Autodesk Inventor part; units mm, degrees
ref_plane "YZ Plane" through (0, 0, 0) normal (1, 0, 0) x (0, 1, 0)
ref_plane "XZ Plane" through (0, 0, 0) normal (0, 1, 0) x (-1, 0, 0)
ref_plane "XY Plane" through (0, 0, 0) normal (0, 0, 1) x (1, 0, 0)
sketch "Sketch1" plane through (0, 0, 0) normal (0, 0, 1) x (1, 0, 0)
  line L0 (323.3438, -62.5) -> (393.7095, -62.5)
  arc A0 (323.3438, -62.5) -> (278.3438, -107.5) centre (323.3438, -107.5) ccw
  line L1 (278.3438, -115) -> (278.3438, -107.5)
  arc A1 (273.3438, -120) -> (278.3438, -115) centre (273.3438, -115) ccw
  line L2 (149.8438, -120) -> (273.3438, -120)
  arc A2 (442.4011, -101.1364) -> (393.7095, -62.5) centre (393.7095, -112.5) ccw
  arc A3 (442.4011, -101.1364) -> (447.2702, -105) centre (447.2702, -100) ccw
  line L3 (453.1438, -105) -> (447.2702, -105)
  arc A4 (453.1438, -105) -> (468.1438, -90) centre (453.1438, -90) ccw
  line L4 (468.1438, 90) -> (468.1438, -90)
  arc A5 (468.1438, 90) -> (453.1438, 105) centre (453.1438, 90) ccw
  line L5 (447.2702, 105) -> (453.1438, 105)
  arc A6 (447.2702, 105) -> (442.4011, 101.1364) centre (447.2702, 100) ccw
  arc A7 (393.7095, 62.5) -> (442.4011, 101.1364) centre (393.7095, 112.5) ccw
  line L6 (393.7095, 62.5) -> (323.3438, 62.5)
  arc A8 (278.3438, 107.5) -> (323.3438, 62.5) centre (323.3438, 107.5) ccw
  line L7 (278.3438, 107.5) -> (278.3438, 115)
  arc A9 (278.3438, 115) -> (273.3438, 120) centre (273.3438, 115) ccw
  line L8 (273.3438, 120) -> (149.8438, 120)
  arc A10 (149.8438, 120) -> (144.8438, 115) centre (149.8438, 115) ccw
  line L9 (144.8438, 115) -> (144.8438, 107.5)
  arc A11 (124.8438, 87.5) -> (144.8438, 107.5) centre (124.8438, 107.5) ccw
  line L10 (106.6438, 87.5) -> (124.8438, 87.5)
  arc A12 (106.6438, 87.5) -> (101.6438, 82.5) centre (106.6438, 82.5) ccw
  line L11 (101.6438, 82.5) -> (101.6438, 63.25)
  arc A13 (96.6438, 58.25) -> (101.6438, 63.25) centre (96.6438, 63.25) ccw
  line L12 (91.6516, 58.25) -> (96.6438, 58.25)
  arc A14 (91.6516, 58.25) -> (85.6702, 54.8864) centre (91.6516, 51.25) ccw
  arc A15 (62.0674, 54.8864) -> (85.6702, 54.8864) centre (73.8688, 62.0613) ccw
  arc A16 (62.0674, 54.8864) -> (56.0861, 58.25) centre (56.0861, 51.25) ccw
  line L13 (56.0861, 58.25) -> (45.5938, 58.25)
  arc A17 (40.5938, 63.25) -> (45.5938, 58.25) centre (45.5938, 63.25) ccw
  line L14 (40.5938, 82.5) -> (40.5938, 63.25)
  arc A18 (40.5938, 82.5) -> (35.5938, 87.5) centre (35.5938, 82.5) ccw
  line L15 (10.1649, 87.5) -> (35.5938, 87.5)
  arc A19 (10.1649, 87.5) -> (5.2408, 83.3682) centre (10.1649, 82.5) ccw
  line L16 (-2.4062, 40) -> (5.2408, 83.3682)
  line L17 (-2.4062, -40) -> (-2.4062, 40)
  line L18 (-2.4062, -40) -> (5.2408, -83.3682)
  arc A20 (5.2408, -83.3682) -> (10.1649, -87.5) centre (10.1649, -82.5) ccw
  line L19 (35.5938, -87.5) -> (10.1649, -87.5)
  arc A21 (35.5938, -87.5) -> (40.5938, -82.5) centre (35.5938, -82.5) ccw
  line L20 (40.5938, -63.25) -> (40.5938, -82.5)
  arc A22 (45.5938, -58.25) -> (40.5938, -63.25) centre (45.5938, -63.25) ccw
  line L21 (56.0861, -58.25) -> (45.5938, -58.25)
  arc A23 (56.0861, -58.25) -> (62.0674, -54.8864) centre (56.0861, -51.25) ccw
  arc A24 (85.6702, -54.8864) -> (62.0674, -54.8864) centre (73.8688, -62.0613) ccw
  arc A25 (85.6702, -54.8864) -> (91.6516, -58.25) centre (91.6516, -51.25) ccw
  line L22 (91.6516, -58.25) -> (96.6438, -58.25)
  arc A26 (101.6438, -63.25) -> (96.6438, -58.25) centre (96.6438, -63.25) ccw
  line L23 (101.6438, -82.5) -> (101.6438, -63.25)
  arc A27 (101.6438, -82.5) -> (106.6438, -87.5) centre (106.6438, -82.5) ccw
  line L24 (106.6438, -87.5) -> (124.8438, -87.5)
  arc A28 (144.8438, -107.5) -> (124.8438, -87.5) centre (124.8438, -107.5) ccw
  line L25 (144.8438, -115) -> (144.8438, -107.5)
  arc A29 (144.8438, -115) -> (149.8438, -120) centre (149.8438, -115) ccw
  line L26 (216.1977, -168) -> (216.1977, 168)
  line L27 (109.0517, -62.5) -> (38.686, -62.5)
  arc A30 (154.0517, -107.5) -> (109.0517, -62.5) centre (109.0517, -107.5) ccw
  line L28 (154.0517, -115) -> (154.0517, -107.5)
  arc A31 (154.0517, -115) -> (159.0517, -120) centre (159.0517, -115) ccw
  line L29 (282.5517, -120) -> (159.0517, -120)
  arc A32 (38.686, -62.5) -> (-10.0056, -101.1364) centre (38.686, -112.5) ccw
  arc A33 (-14.8747, -105) -> (-10.0056, -101.1364) centre (-14.8747, -100) ccw
  line L30 (-20.7483, -105) -> (-14.8747, -105)
  arc A34 (-35.7483, -90) -> (-20.7483, -105) centre (-20.7483, -90) ccw
  line L31 (-35.7483, 90) -> (-35.7483, -90)
  arc A35 (-20.7483, 105) -> (-35.7483, 90) centre (-20.7483, 90) ccw
  line L32 (-14.8747, 105) -> (-20.7483, 105)
  arc A36 (-10.0056, 101.1364) -> (-14.8747, 105) centre (-14.8747, 100) ccw
  arc A37 (-10.0056, 101.1364) -> (38.686, 62.5) centre (38.686, 112.5) ccw
  line L33 (38.686, 62.5) -> (109.0517, 62.5)
  arc A38 (109.0517, 62.5) -> (154.0517, 107.5) centre (109.0517, 107.5) ccw
  line L34 (154.0517, 107.5) -> (154.0517, 115)
  arc A39 (159.0517, 120) -> (154.0517, 115) centre (159.0517, 115) ccw
  line L35 (159.0517, 120) -> (282.5517, 120)
  arc A40 (287.5517, 115) -> (282.5517, 120) centre (282.5517, 115) ccw
  line L36 (287.5517, 115) -> (287.5517, 107.5)
  arc A41 (287.5517, 107.5) -> (307.5517, 87.5) centre (307.5517, 107.5) ccw
  line L37 (325.7517, 87.5) -> (307.5517, 87.5)
  arc A42 (330.7517, 82.5) -> (325.7517, 87.5) centre (325.7517, 82.5) ccw
  line L38 (330.7517, 82.5) -> (330.7517, 63.25)
  arc A43 (330.7517, 63.25) -> (335.7517, 58.25) centre (335.7517, 63.25) ccw
  line L39 (340.7439, 58.25) -> (335.7517, 58.25)
  arc A44 (346.7253, 54.8864) -> (340.7439, 58.25) centre (340.7439, 51.25) ccw
  arc A45 (346.7253, 54.8864) -> (370.3281, 54.8864) centre (358.5267, 62.0613) ccw
  arc A46 (376.3094, 58.25) -> (370.3281, 54.8864) centre (376.3094, 51.25) ccw
  line L40 (376.3094, 58.25) -> (386.8017, 58.25)
  arc A47 (386.8017, 58.25) -> (391.8017, 63.25) centre (386.8017, 63.25) ccw
  line L41 (391.8017, 82.5) -> (391.8017, 63.25)
  arc A48 (396.8017, 87.5) -> (391.8017, 82.5) centre (396.8017, 82.5) ccw
  line L42 (422.2306, 87.5) -> (396.8017, 87.5)
  arc A49 (427.1547, 83.3682) -> (422.2306, 87.5) centre (422.2306, 82.5) ccw
  line L43 (434.8017, 40) -> (427.1547, 83.3682)
  line L44 (434.8017, -40) -> (434.8017, 40)
  line L45 (434.8017, -40) -> (427.1547, -83.3682)
  arc A50 (422.2306, -87.5) -> (427.1547, -83.3682) centre (422.2306, -82.5) ccw
  line L46 (396.8017, -87.5) -> (422.2306, -87.5)
  arc A51 (391.8017, -82.5) -> (396.8017, -87.5) centre (396.8017, -82.5) ccw
  line L47 (391.8017, -63.25) -> (391.8017, -82.5)
  arc A52 (391.8017, -63.25) -> (386.8017, -58.25) centre (386.8017, -63.25) ccw
  line L48 (376.3094, -58.25) -> (386.8017, -58.25)
  arc A53 (370.3281, -54.8864) -> (376.3094, -58.25) centre (376.3094, -51.25) ccw
  arc A54 (370.3281, -54.8864) -> (346.7253, -54.8864) centre (358.5267, -62.0613) ccw
  arc A55 (340.7439, -58.25) -> (346.7253, -54.8864) centre (340.7439, -51.25) ccw
  line L49 (340.7439, -58.25) -> (335.7517, -58.25)
  arc A56 (335.7517, -58.25) -> (330.7517, -63.25) centre (335.7517, -63.25) ccw
  line L50 (330.7517, -82.5) -> (330.7517, -63.25)
  arc A57 (325.7517, -87.5) -> (330.7517, -82.5) centre (325.7517, -82.5) ccw
  line L51 (325.7517, -87.5) -> (307.5517, -87.5)
  arc A58 (307.5517, -87.5) -> (287.5517, -107.5) centre (307.5517, -107.5) ccw
  line L52 (287.5517, -115) -> (287.5517, -107.5)
  arc A59 (282.5517, -120) -> (287.5517, -115) centre (282.5517, -115) ccw
  point P0 (0, 0)
  point P1 (432.3955, 0)
extrude "Extrusion1" add sketch "Sketch1" against normal blind 5 contours A0 L1 A1 L2 L26 L8 A9 L7 A8 L6 A43 L39 A44 A45 A46 L40 A47 A7 L43 L44 L45 A2 L0 A52 L48 A53 A54 A55 L49 A56 | A56 L49 A55 A54 A53 L48 A52 L0 | L45 L44 L43 A7 A6 L5 A5 L4 A4 L3 A3 A2 | L2 A31 L28 A30 L27 A26 L22 A25 A24 A23 L21 A22 A32 L18 L17 L16 A37 L33 A17 L13 A16 A15 A14 L12 A13 A38 L34 A39 L8 L26 | A47 L40 A46 A45 A44 L39 A43 L6 | L27 A22 L21 A23 A24 A25 L22 A26 | A13 L12 A14 A15 A16 L13 A17 L33 | A32 A33 L30 A34 L31 A35 L32 A36 A37 L16 L17 L18
properties part number "my_base"
Geometry: final body of the model. Coordinates: model frame, mm. A direction names the side the tool comes from. Round coordinates to 2 decimals unless told otherwise and drop trailing zeros. Order: outer loops, then holes, each group sorted by start corner. A loop starts at its lowest first (then second) coordinate and runs counter-clockwise, first axis right, second up. Notation, with made-up numbers: (86, -35) -> (115, -35) arc R12 ccw to (115, -18) -> close; hole circle Ø9 at (41, -24.5). An arc over 180 degrees is marked (long way). Use CSV: the item, a comma, the result in double quotes. Start each with the question number.
1) Section C-C (x = -4.5). Return the cut outline in (y, z).
2) First-contact query: pin 1 Ø1.5 at (y, z) = (-112, -1.5) entering from -X; pin 2 Ø1.5 at (x, z) = (-17, -3) entering from -Y; pin 3 Ø1.5 at (x, z) = (368.5, -3) entering from -Y. Flat tips, straight axial feed; report the tip coordinate or a pass-through.
3) Section B-B (x = 355.5). Return the cut outline in (y, z).
4) Draft query along X for faces 1 (the face through (213, 2, -5)), 2 (the face through (-31.47, -100.49, -2.46)), 3 (the face through (424.419, 73.042, -2.465)). Return one class per face: +X half, -X half, draft (parallel to the pull), parting line (faces both ways), or undercut.
5) Section A-A (y = 85). Return the cut outline in (x, z).
6) Material intervals for line 1 along Y through (x, z) = (107, -2.65); line 2 along X through (y, z) = (107.5, -3.45); line 3 along X through (y, z) = (-67, -1.75), sorted ascending. Write a range as from..to.
7) Set-up query: faces 4 (the face through (213, 2, 0)), 5 (the face through (141.22, -76.03, -2.46)), 6 (the face through (140.52, 75.33, -2.46)). Return all of +Z, -Z, +X, -X, +Y, -Y with unobstructed straight access to the full face (end or side cutting, diameter ignored); none if empty.
Returned:
1,outline,"(-87.3, -5) -> (87.3, -5) -> (87.3, 0) -> (-87.3, 0) -> close"
2,pin 1,"stops at x = 154.05"
2,pin 2,"stops at y = -105"
2,pin 3,"stops at y = -62.5"
3,outline,"(-62.5, -5) -> (62.5, -5) -> (62.5, 0) -> (-62.5, 0) -> close"
4,face 1,"draft"
4,face 2,"-X half"
4,face 3,"undercut"
5,outline,"(-35.75, -5) -> (-3.07, -5) -> (-3.07, 0) -> (-35.75, 0) -> close; (148.02, -5) -> (284.37, -5) -> (284.37, 0) -> (148.02, 0) -> close; (435.47, -5) -> (468.14, -5) -> (468.14, 0) -> (435.47, 0) -> close"
6,line 1,"y = -62.5..62.5"
6,line 2,"x = 154.05..278.34"
6,line 3,"x = -35.75..17.96, 128.67..303.73, 414.44..468.14"
7,face 4,"+Z, +X, -X, +Y, -Y"
7,face 5,"+Z, -Z, -Y"
7,face 6,"+Z, -Z, +Y"
